Read the model definition and answer for the solid it produces. Units are mm, in the model's axes. Face numbers are marked on the shaded views. A direction names the side the tool comes from. Coordinates: 2 decimals unless noted, no trailing zeros. Loops run counter-clockwise (first coordinate to the right, second up) from the corner with the lowest first, then second, coordinate; pieces in that order, holes last. Notation, with made-up numbers: (-39, 70.25) -> (-3, 70.25) arc R28 ccw to (-3, 108.25) -> close; hole circle Ø9 at (-22.75, 10). An arc over 180 degrees is marked (long way). Answer as a JSON object with one key per item and string values. Group by question number.
1) Determine the mould class of the marked faces 1, 2 and 3 for opening direction Y: released by +Y, released by -Y, zero draft, split by the parting line, or undercut.
2) Section D-D, the plane z = 50 is taken. Give the vertices of the cut face in (x, y), plus the area to 3 significant figures.
3) Flat-ended cylindrical pins translate along their axes: P1, Ø2.5, axis at y = -119.5, z = 2.5, coming from the -X side; P2, Ø2, axis at y = -213.5, z = 30, coming from the -X side; P3, Ø3, axis at x = -241.5, y = -260, coming from the -Z side; P4, Ø4, axis at y = -279.5, z = 11, coming from the +X side. Find the tip coordinate at first contact, or state that the pin passes through.
4) Section A-A, the plane x = -333.5 is taken. Give the vertices of the cut face in (y, z) (3 decimals), plus the area to 3 significant figures.
5) Consider probe 1 along Z at (x, y) = (-218.5, -172); probe 2 along Y at (x, z) = (-178.5, 39); probe 3 along X at (y, z) = (-16, 32). Determine where each line is inside the solid, lowest interval first. Write a range as [from, to].
6) Section B-B, the plane y = -129 is taken. Give the vertices of the cut face in (x, z).
7) Which of the six approach directions +Z, -Z, +X, -X, +Y, -Y give full straight-line access (tool end or side, diameter ignored) to the marked faces 4, 5 and 6?
8) Section C-C, the plane x = -169 is taken. Give the vertices of the cut face in (y, z).
from build123d import *

# Parameters (mm, degrees)
F0_W     = 419.1
F0_H     = 73.66
F1_DEPTH = 323.85
F2_W     = 313.69
F2_H     = 63.5
F3_DEPTH = 304.8
F4_W     = 313.69
F4_H     = 63.5
F5_DEPTH = 109.22
F7_DEPTH = 323.85
F8_W     = 177.8
F8_H     = 177.8
F9_DEPTH = 73.661


with BuildPart() as f1:
    # F0 (on Front) → F1 (new body)
    with BuildSketch(Plane.XZ):
        with Locations((-209.55, 36.83)):
            Rectangle(F0_W, F0_H)
    extrude(amount=F1_DEPTH)

    # F2 (on face) → F3 (cut)
    with BuildSketch(Plane(origin=(-419.1, 0, 0), x_dir=(0, -1, 0), z_dir=(-1, 0, 0))):
        with Locations((161.925, 36.83)):
            Rectangle(F2_W, F2_H)
    extrude(amount=-F3_DEPTH, mode=Mode.SUBTRACT)

    # F4 (on face) → F5 (cut)
    with BuildSketch(Plane.YZ):
        with Locations((-161.925, 36.83)):
            Rectangle(F4_W, F4_H)
    extrude(amount=-F5_DEPTH, mode=Mode.SUBTRACT)

    # F6 (on face) → F7 (cut, through all)
    with BuildSketch(Plane.XZ):
        Polygon((-19.000666, 61.750006), (-16.534498, 55.898466), (-10.233832, 55.10846), (-6.399334, 60.169994), (-8.865502, 66.021534), (-15.166168, 66.81154), align=None)
    extrude(amount=F7_DEPTH, mode=Mode.SUBTRACT)

    # F8 (on face) → F9 (cut, through all)
    with BuildSketch(Plane(origin=(0, 0, 0), x_dir=(1, 0, 0), z_dir=(0, 0, -1))):
        with Locations((-330.2, 161.925)):
            Rectangle(F8_W, F8_H)
    extrude(amount=-F9_DEPTH, mode=Mode.SUBTRACT)


solid = f1.part
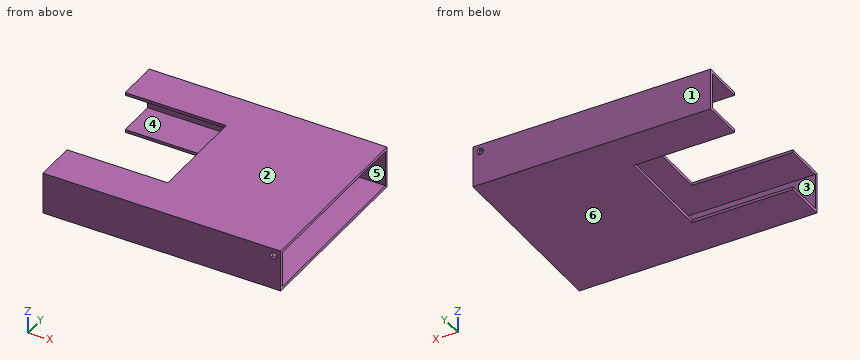
Determined:
{
 "1": {"face 1": "released by +Y", "face 2": "zero draft", "face 3": "undercut"},
 "2": {"outline": "(-419.1, -323.85) -> (0, -323.85) -> (0, -318.77) -> (-109.22, -318.77) -> (-109.22, -5.08) -> (0, -5.08) -> (0, 0) -> (-419.1, 0) -> (-419.1, -5.08) -> (-114.3, -5.08) -> (-114.3, -318.77) -> (-419.1, -318.77) -> close", "area": "5,850 mm²"},
 "3": {"P1": "x = -241.3", "P2": "x = -114.3", "P3": "z = 0", "P4": "x = -109.22"},
 "4": {"outline": "(-323.85, 0) -> (-250.825, 0) -> (-250.825, 5.08) -> (-318.77, 5.08) -> (-318.77, 68.58) -> (-250.825, 68.58) -> (-250.825, 73.66) -> (-323.85, 73.66) -> close; (-73.025, 0) -> (0, 0) -> (0, 73.66) -> (-73.025, 73.66) -> (-73.025, 68.58) -> (-5.08, 68.58) -> (-5.08, 5.08) -> (-73.025, 5.08) -> close", "area": "2,130 mm²"},
 "5": {"probe 1": "[0, 5.08], [68.58, 73.66]", "probe 2": "[-323.85, -318.77], [-5.08, 0]", "probe 3": "[-114.3, -109.22]"},
 "6": {"outline": "(-241.3, 0) -> (0, 0) -> (0, 5.08) -> (-109.22, 5.08) -> (-109.22, 68.58) -> (0, 68.58) -> (0, 73.66) -> (-241.3, 73.66) -> (-241.3, 68.58) -> (-114.3, 68.58) -> (-114.3, 5.08) -> (-241.3, 5.08) -> close"},
 "7": {"face 4": "-X", "face 5": "+X", "face 6": "-Z, +X, -X, +Y, -Y"},
 "8": {"outline": "(-323.85, 0) -> (0, 0) -> (0, 73.66) -> (-323.85, 73.66) -> close; hole (-318.77, 5.08) -> (-5.08, 5.08) -> (-5.08, 68.58) -> (-318.77, 68.58) -> close"}
}
